Build history of the part. All positions in model axes, mm. Face numbers are marked on the shaded views. A direction names the side the tool comes from. Round coordinates to 2 decimals unless told otherwise and drop trailing zeros. Loops run counter-clockwise (first coordinate to the right, second up) from the corner with the lowest first, then second, coordinate; pieces in that order, holes last. Notation, with made-up numbers: (30, 19) - (56, 19) arc R11 cw to (56, 23) - close; hole circle Ø8 at (-17.75, 0). An arc over 180 degrees is marked (long way). Use one line per item in the form item = value. Start each with the question number.
Q1. Drill centre lines: line 1 (Z direction, x = 607, y = -747); line 2 (X direction, y = -713, z = -557); line 3 (Z direction, x = 916, y = 356). Where is each one in solid material? Low to high.
Q2. Saw through at B-B (x = 266). Give the cut face in (y, z), then the cut area to 3 significant figures.
Q3. Saw through at A-A (y = -720). Give the cut face in (x, z), then the cut area to 3 significant figures.
Q4. 3-axis set-ups, long thin cutter, end or side, ignore diameter. For the marked faces 1, 2 and 3: which of +Z, -Z, +X, -X, +Y, -Y reach the whole face in a straight line?
Q5. Pin check, flat tips, straight feed: pin 1 (12 mm diameter, centred on x = 1163.5, y = 457, fed in from +Z); pin 2 (2 mm diameter, centred on y = 245, z = -247.5, fed in from +X); pin 3 (6 mm diameter, centred on x = 672, y = 573, fed in from +Z). Stop position of each tip, or through.
Q6. Saw through at C-C (z = -436.5). Give the cut face in (x, y).
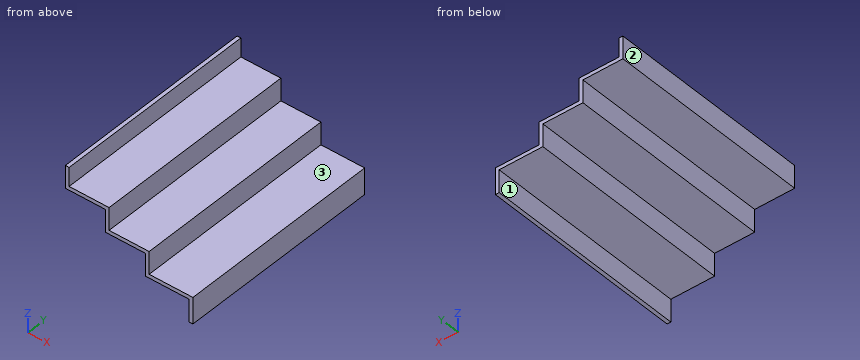
```python
from build123d import *

# Parameters (mm, degrees)
F0_W      = 2082.8
F0_H      = 190.5
F0_H_2    = 38.1
F1_DEPTH  = 38.1
F2_DEPTH  = 444.5
F3_W      = 38.1
F3_H      = 2082.8
F4_DEPTH  = 266.7
F5_W      = 2082.8
F5_H      = 38.1
F6_DEPTH  = 444.5
F7_W      = 38.1
F7_H      = 2082.8
F8_DEPTH  = 266.7
F9_W      = 2082.8
F9_H      = 38.1
F10_DEPTH = 482.6
F11_W     = 38.1
F11_H     = 2082.8
F12_DEPTH = 266.7


with BuildPart() as f1:
    # F0 (on Right) → F1 (new body)
    with BuildSketch(Plane.YZ):
        with Locations((0, 19.05)):
            Rectangle(F0_W, F0_H)
        with Locations((0, -95.25)):
            Rectangle(F0_W, F0_H_2)
    extrude(amount=F1_DEPTH)

    # F0 (on Right) → F2 (join)
    with BuildSketch(Plane.YZ):
        with Locations((0, -95.25)):
            Rectangle(F0_W, F0_H_2)
    extrude(amount=F2_DEPTH)

    # F3 (on face) → F4 (join)
    with BuildSketch(Plane.XY.offset(-76.2)):
        with Locations((425.45, 0)):
            Rectangle(F3_W, F3_H)
    extrude(amount=-F4_DEPTH)

    # F5 (on face) → F6 (join)
    with BuildSketch(Plane(origin=(406.4, 0, 0), x_dir=(0, -1, 0), z_dir=(-1, 0, 0))):
        with Locations((0, -323.85)):
            Rectangle(F5_W, F5_H)
    extrude(amount=-F6_DEPTH)

    # F7 (on face) → F8 (join)
    with BuildSketch(Plane.XY.offset(-304.8)):
        with Locations((831.85, 0)):
            Rectangle(F7_W, F7_H)
    extrude(amount=-F8_DEPTH)

    # F9 (on face) → F10 (join)
    with BuildSketch(Plane(origin=(812.8, 0, 0), x_dir=(0, -1, 0), z_dir=(-1, 0, 0))):
        with Locations((0, -552.45)):
            Rectangle(F9_W, F9_H)
    extrude(amount=-F10_DEPTH)

    # F11 (on face) → F12 (join)
    with BuildSketch(Plane.XY.offset(-533.4)):
        with Locations((1276.35, 0)):
            Rectangle(F11_W, F11_H)
    extrude(amount=-F12_DEPTH)


solid = f1.part
```
Report:
q1.line_1 = -342.9 to -304.8
q1.line_2 = 812.8 to 1295.4
q1.line_3 = -571.5 to -533.4
q2.outline = (-1041.4, -114.3) - (1041.4, -114.3) - (1041.4, -76.2) - (-1041.4, -76.2) - close
q2.area = 79,400 mm²
q3.outline = (0, -114.3) - (406.4, -114.3) - (406.4, -342.9) - (812.8, -342.9) - (812.8, -571.5) - (1257.3, -571.5) - (1257.3, -800.1) - (1295.4, -800.1) - (1295.4, -533.4) - (850.9, -533.4) - (850.9, -304.8) - (444.5, -304.8) - (444.5, -76.2) - (38.1, -76.2) - (38.1, 114.3) - (0, 114.3) - close
q3.area = 82,700 mm²
q4.face_1 = -Z, -X, +Y, -Y
q4.face_2 = +Z, -Z, -X, +Y, -Y
q4.face_3 = +Z, +X, +Y, -Y
q5.pin_1 = -533.4
q5.pin_2 = 444.5
q5.pin_3 = -304.8
q6.outline = (812.8, -1041.4) - (850.9, -1041.4) - (850.9, 1041.4) - (812.8, 1041.4) - close
